```python
from build123d import *

# Parameters (mm, degrees)
SKETCH_1_R      = 1.5
EXTRUDE_1_DEPTH = 7
SKETCH_3_R      = 1.7
SKETCH_3_R_2    = 2
EXTRUDE_2_DEPTH = 4


with BuildPart() as part:
    # Sketch 1 → Extrude 1 (new body)
    with BuildSketch(Plane(origin=(0, 0, 0), x_dir=(1, 0, 0), z_dir=(0, 1, 0))):
        with BuildLine():
            ThreePointArc((-24.592495152, -18.040487305), (-21.566756826, -21.566756826), (-18.040487305, -24.592495152))
            ThreePointArc((-18.040487305, -24.592495152), (-13.847079195, -23.948035364), (-14.491538983, -19.754627253))
            ThreePointArc((-14.491538983, -19.754627253), (-17.324116139, -17.324116139), (-19.754627253, -14.491538983))
            ThreePointArc((-19.754627253, -14.491538983), (-23.948035364, -13.847079195), (-24.592495152, -18.040487305))
        make_face()
        with Locations(Location((-19.445436483, -19.445436483, 0), (0, 0, 270))):
            Circle(SKETCH_1_R, mode=Mode.SUBTRACT)
    extrude(amount=EXTRUDE_1_DEPTH)

    # Sketch 2 → Cut-Revolve 1 (revolve, cut)
    with BuildSketch(Plane(origin=(-19.445436483, 0, 0), x_dir=(0, 0, -1), z_dir=(1, 0, 0))):
        Polygon((-19.445436483, 7), (-21.945436483, 7), (-20.695436483, 4.5), (-19.445436483, 4.5), align=None)
    revolve(axis=Axis((-19.445436483, 7, 19.445436483), (0, -1, 0)), mode=Mode.SUBTRACT)

    # Sketch 3 → Extrude 2 (add)
    with BuildSketch(Plane.XZ):
        with Locations(Location((-15.969331282, 22.388176755, 0), (0, 0, 90))):
            Circle(SKETCH_3_R)
        with Locations(Location((-22.388176755, 15.969331282, 0), (0, 0, 90))):
            Circle(SKETCH_3_R_2)
    extrude(amount=EXTRUDE_2_DEPTH)


solid = part.part
```
Check sheet for the modelled part. Datum: model origin and axes. Units: mm. A direction names the side the tool comes from. Coordinates: 2 decimals unless noted, no trailing zeros. Write each loop counter-clockwise with the first axis right and the second up, starting at its lowest first coordinate (ties: lowest second). Pieces come first, ordered by that corner, then holes. Notation, with made-up numbers: M -19,31 L -15,31 A22 cw -15,50 Z; hole C -27.75,48 d10. An arc over 180 degrees is marked long. Write item = value, one per line. Start each with the question number.
1. Thickness scan on probe 1 along Y at (x, z) = (-17.5, 17.5); probe 2 along Z at (x, y) = (-20, 5.25); probe 3 along X at (y, z) = (0.25, 20). Record the ranges inside material, lowest first.
2. Sectioned sample at B-B (y = -2.75). Record the cut outline in (x, z).
3. Go/stop test with a flat-tipped pin: pin 1 (2 mm diameter, centred on x = -16.5, z = 17.5, fed in from -Y). Record where the tip stops, or that it passes through.
4. Sectioned sample at A-A (y = 4.5). Record the cut outline in (x, z).
5. Tool access check on faces 1 (the cylindrical face through (-20.436, -1.972, 15.536)), 2 (the flat face through (-22, -4, 16)). Record the directions out of +Z, -Z, +X, -X, +Y, -Y that give a thin tool (end or side, any length) a straight path to the whole face; none if there is none.
6. Sectioned sample at D-D (x = -15.5). Record the cut outline in (y, z), then the cut area to 3 significant figures.
7. Sectioned sample at C-C (z = 14.75). Record the cut outline in (x, y).
8. Mould release check, pull along Z, two halves, no side actions. Record for faces 3 (the cylindrical face through (-21.613, 3.451, 21.521)), 4 (the cylindrical face through (-18.995, 2.465, 20.876)), 5 (the cylindrical face through (-23.894, 3.451, 13.809)), 6 (the flat face through (-19, 7, 16)): pulls with the +Z half, pulls with the -Z half, needs draft (parallel to the pull), parting line crosses it, or undercut.
The answers:
q1.probe_1 = 0 to 7
q1.probe_2 = 14.2 to 17.92, 20.97 to 23.03
q1.probe_3 = -23.03 to -20.84, -18.05 to -14.2
q2.outline = C -22.39,15.97 d4; C -15.97,22.39 d3.4
q3.pin_1 = 0
q4.outline = M -24.59,18.04 A3 ccw -19.75,14.49 A24.5 cw -14.49,19.75 A3 ccw -18.04,24.59 A30.5 ccw Z; hole C -19.45,19.45 d3
q5.face_1 = -Y
q5.face_2 = +Z, -Z, +X, -X, -Y
q6.outline = M -4,20.75 L 0,20.75 L 0,18.97 L 7,18.97 L 7,25.07 L 0,25.07 L 0,24.02 L -4,24.02 Z
q6.area = 55.8 mm²
q7.outline = M -24.76,0 L -23.97,0 L -23.97,-4 L -20.8,-4 L -20.8,0 L -19.56,0 L -19.56,7 L -24.76,7 Z
q8.face_3 = pulls with the +Z half
q8.face_4 = undercut
q8.face_5 = parting line crosses it
q8.face_6 = needs draft
